Verification items for the finished model (mm, model axes). Give positions to 0.01 mm unless a question says otherwise; leave off trailing zeros. Order: outer loops, then holes, each group sorted by start corner. A loop starts at its lowest first (then second) coordinate and runs counter-clockwise, first axis right, second up.
(1) Scan lines: L1, parallel to X at y = 8, z = -0.75; L2, parallel to Y at x = 124, z = -2.75; L3, parallel to Z at x = 189, y = 13.25. Record each from-to range of solid material in increasing order.
(2) Sectioned sample at B-B on x = 371. Record the cut outline in (y, z), plus the area to 3 significant figures.
(3) Gauge pin test, flat ends, axial feed: pin 1 (0.9 mm diameter, centred on y = 4.5, z = -1.5, fed in from -X); pin 2 (2.5 mm diameter, centred on y = 6, z = -1, fed in from +X); pin 3 (3 mm diameter, centred on x = 175.5, y = 12.5, fed in from -Z). Record the tip position at first contact, or that the pin passes through.
(4) Sectioned sample at C-C on x = 47.5. Record the cut outline in (y, z).
(5) Sectioned sample at A-A on y = 8. Record the cut outline in (x, z), plus the area to 3 significant figures.
```python
from build123d import *

# Parameters (mm, degrees)
EXTRUDE_1_DEPTH     = 396
SKETCH_4_R          = 2.25
CUT_EXTRUDE_3_DEPTH = 2
CHAMFER_1_SIZE      = 2.05
CUT_EXTRUDE_5_DEPTH = 14
CUT_EXTRUDE_6_DEPTH = 14
CUT_EXTRUDE_7_DEPTH = 397.497162663
SKETCH_10_R         = 2.25
CUT_EXTRUDE_8_DEPTH = 397.497162663


with BuildPart() as part:
    # Эскиз1 → Бобышка-Вытянуть1 (new body)
    with BuildSketch(Plane(origin=(0, 0, 0), x_dir=(0, 0, -1), z_dir=(1, 0, 0))):
        with BuildLine():
            Line((0, 0), (0, 15))
            Line((0, 15), (1, 15))
            ThreePointArc((1, 15), (1.707106781, 14.707106781), (2, 14))
            Line((2, 14), (2, 3))
            ThreePointArc((2, 3), (2.292893219, 2.292893219), (3, 2))
            Line((3, 2), (14, 2))
            ThreePointArc((14, 2), (14.707106781, 1.707106781), (15, 1))
            Line((15, 1), (15, 0))
            Line((15, 0), (0, 0))
        make_face()
    extrude(amount=EXTRUDE_1_DEPTH)

    # Эскиз4 → Вырез-Вытянуть3 (cut)
    with BuildSketch(Plane.XZ):
        with Locations(Location((371, -8, 0), (0, 0, 270))):
            Circle(SKETCH_4_R)
        with Locations(Location((198, -8, 0), (0, 0, 270))):
            Circle(SKETCH_4_R)
        with Locations(Location((25, -8, 0), (0, 0, 270))):
            Circle(SKETCH_4_R)
    extrude(amount=-CUT_EXTRUDE_3_DEPTH, mode=Mode.SUBTRACT)

    # Фаска1
    # the kernel refuses this chamfer: 2.05 mm, written as the material it takes off along each edge
    with BuildSketch(Plane(origin=(25, 0, -8), x_dir=(0, 0, -1), z_dir=(-1, 0, 0))) as chamfer_1_piece_1:
        Polygon((2.25 + CHAMFER_1_SIZE, 0), (2.25, -CHAMFER_1_SIZE), (2.25, 0), align=None)
    revolve(axis=Axis((25, 0, -8), (0, -1, 0)), mode=Mode.SUBTRACT)
    with BuildSketch(Plane(origin=(371, 0, -8), x_dir=(0, 0, -1), z_dir=(-1, 0, 0))) as chamfer_1_piece_2:
        Polygon((2.25 + CHAMFER_1_SIZE, 0), (2.25, -CHAMFER_1_SIZE), (2.25, 0), align=None)
    revolve(axis=Axis((371, 0, -8), (0, -1, 0)), mode=Mode.SUBTRACT)
    with BuildSketch(Plane(origin=(198, 0, -8), x_dir=(0, 0, -1), z_dir=(-1, 0, 0))) as chamfer_1_piece_3:
        Polygon((2.25 + CHAMFER_1_SIZE, 0), (2.25, -CHAMFER_1_SIZE), (2.25, 0), align=None)
    revolve(axis=Axis((198, 0, -8), (0, -1, 0)), mode=Mode.SUBTRACT)

    # Эскиз6 → Вырез-Вытянуть5 (cut)
    with BuildSketch(Plane(origin=(396, 0, 0), x_dir=(0, 0, -1), z_dir=(1, 0, 0))):
        Polygon((0, 15), (2, 15), (3, 15), (3, 2), (2, 2), (2, 0), (0, 0), align=None)
    extrude(amount=-CUT_EXTRUDE_5_DEPTH, mode=Mode.SUBTRACT)

    # Эскиз7 → Вырез-Вытянуть6 (cut)
    with BuildSketch(Plane.ZY):
        Polygon((0, 15), (-2, 15), (-3, 15), (-3, 2), (-2, 2), (-2, 0), (0, 0), align=None)
    extrude(amount=-CUT_EXTRUDE_6_DEPTH, mode=Mode.SUBTRACT)

    # Эскиз9 → Вырез-Вытянуть7 (cut, through all)
    with BuildSketch(Plane(origin=(0, 2, 0), x_dir=(1, 0, 0), z_dir=(0, 1, 0))):
        Polygon((0, 2), (0, 7), (5, 2), align=None)
        Polygon((396, 2), (396, 7), (391, 2), align=None)
    extrude(amount=-CUT_EXTRUDE_7_DEPTH, mode=Mode.SUBTRACT)

    # Эскиз10 → Вырез-Вытянуть8 (cut, through all)
    with BuildSketch(Plane(origin=(0, 0, -2), x_dir=(-1, 0, 0), z_dir=(0, 0, -1))):
        with Locations(Location((-72, 8, 0), (0, 0, 90))):
            Circle(SKETCH_10_R)
        with Locations(Location((-110, 8, 0), (0, 0, 90))):
            Circle(SKETCH_10_R)
    extrude(amount=-CUT_EXTRUDE_8_DEPTH, mode=Mode.SUBTRACT)


solid = part.part
```
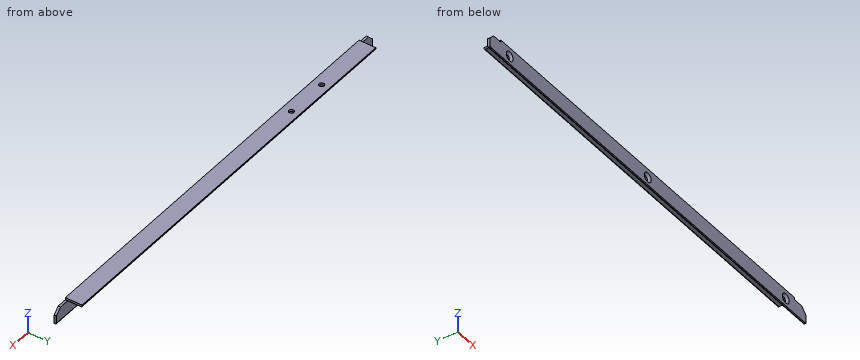
Ans:
1. L1: x = 14 to 69.75, 74.25 to 107.75, 112.25 to 382
1. L2: y = 0 to 2.03
1. L3: z = -2 to 0
2. outline: (0, -15) - (1, -15) arc R1 ccw to (2, -14) - (2, -10.3) - (0, -12.3) - close; (0, -3.7) - (2, -5.7) - (2, -3) arc R1 cw to (3, -2) - (14, -2) arc R1 ccw to (15, -1) - (15, 0) - (0, 0) - close
2. area: 42.6 mm2
3. pin 1: stops at x = 14
3. pin 2: stops at x = 382
3. pin 3: stops at z = -2
4. outline: (0, -15) - (1, -15) arc R1 ccw to (2, -14) - (2, -3) arc R1 cw to (3, -2) - (14, -2) arc R1 ccw to (15, -1) - (15, 0) - (0, 0) - close
5. outline: (14, -2) - (69.75, -2) - (69.75, 0) - (14, 0) - close; (74.25, -2) - (107.75, -2) - (107.75, 0) - (74.25, 0) - close; (112.25, -2) - (382, -2) - (382, 0) - (112.25, 0) - close
5. area: 718 mm2
